```python
from build123d import *

# Parameters (mm, degrees)
SKETCH1_R           = 19.075
SKETCH1_R_2         = 2.675
BOSS_EXTRUDE1_DEPTH = 2.54
BOSS_EXTRUDE2_START = -2.54
SKETCH2_R           = 2.675
SKETCH2_R_2         = 2
BOSS_EXTRUDE2_DEPTH = 2.54
CUT_EXTRUDE1_DEPTH  = 43.502371699


with BuildPart() as part:
    # Sketch1 → Boss-Extrude1 (new body)
    with BuildSketch(Plane(origin=(0, 0, 0), x_dir=(0, 0, -1), z_dir=(1, 0, 0))):
        with BuildLine():
            Line((-30, 26.457513111), (-30, -26.457513111))
            ThreePointArc((-30, -26.457513111), (-28.284271247, -28.284271247), (-26.457513111, -30))
            Line((-26.457513111, -30), (26.457513111, -30))
            ThreePointArc((26.457513111, -30), (28.284271247, -28.284271247), (30, -26.457513111))
            Line((30, -26.457513111), (30, 26.457513111))
            ThreePointArc((30, 26.457513111), (28.284271247, 28.284271247), (26.457513111, 30))
            Line((26.457513111, 30), (-26.457513111, 30))
            ThreePointArc((-26.457513111, 30), (-28.284271247, 28.284271247), (-30, 26.457513111))
        make_face()
        Circle(SKETCH1_R, mode=Mode.SUBTRACT)
        with Locations((-23.425, -23.425)):
            Circle(SKETCH1_R_2, mode=Mode.SUBTRACT)
        with Locations((23.425, -23.425)):
            Circle(SKETCH1_R_2, mode=Mode.SUBTRACT)
        with Locations((23.425, 23.425)):
            Circle(SKETCH1_R_2, mode=Mode.SUBTRACT)
        with Locations((-23.425, 23.425)):
            Circle(SKETCH1_R_2, mode=Mode.SUBTRACT)
    extrude(amount=BOSS_EXTRUDE1_DEPTH)

    # Sketch2 → Boss-Extrude2 (add)
    # profile 1 of 4: a face of its own
    with BuildSketch(Plane(origin=(2.54, 0, 0), x_dir=(0, 0, -1), z_dir=(1, 0, 0)).offset(BOSS_EXTRUDE2_START)):
        with Locations((-23.425, -23.425)):
            Circle(SKETCH2_R)
        with Locations((-23.425, -23.425)):
            Circle(SKETCH2_R_2, mode=Mode.SUBTRACT)
    # profile 2 of 4: a face of its own
    with BuildSketch(Plane(origin=(2.54, 0, 0), x_dir=(0, 0, -1), z_dir=(1, 0, 0)).offset(BOSS_EXTRUDE2_START)):
        with Locations((23.425, 23.425)):
            Circle(SKETCH2_R)
        with Locations((23.425, 23.425)):
            Circle(SKETCH2_R_2, mode=Mode.SUBTRACT)
    # profile 3 of 4: a face of its own
    with BuildSketch(Plane(origin=(2.54, 0, 0), x_dir=(0, 0, -1), z_dir=(1, 0, 0)).offset(BOSS_EXTRUDE2_START)):
        with Locations((23.425, -23.425)):
            Circle(SKETCH2_R)
        with Locations((23.425, -23.425)):
            Circle(SKETCH2_R_2, mode=Mode.SUBTRACT)
    # profile 4 of 4: a face of its own
    with BuildSketch(Plane(origin=(2.54, 0, 0), x_dir=(0, 0, -1), z_dir=(1, 0, 0)).offset(BOSS_EXTRUDE2_START)):
        with Locations((-23.425, 23.425)):
            Circle(SKETCH2_R)
        with Locations((-23.425, 23.425)):
            Circle(SKETCH2_R_2, mode=Mode.SUBTRACT)
    extrude(amount=BOSS_EXTRUDE2_DEPTH)

    # Sketch3 → Cut-Extrude1 (cut, through all)
    with BuildSketch(Plane(origin=(2.54, 0, 0), x_dir=(0, 0, -1), z_dir=(1, 0, 0))):
        Polygon((-14.125, 30), (-14.125, 12.819516372), (16.436338552, -9.68), (30, -9.68), (30, 30), align=None)
    extrude(amount=-CUT_EXTRUDE1_DEPTH, mode=Mode.SUBTRACT)


solid = part.part
```
The model under review builds one solid part; all positions refer to its coordinate system, in mm. A direction names the side the tool comes from. Round coordinates to 2 decimals unless told otherwise and drop trailing zeros. Write each loop counter-clockwise with the first axis right and the second up, starting at its lowest first coordinate (ties: lowest second). Pieces come first, ordered by that corner, then holes.
(1) We need section B-B on x = 2.15. Give the boundary of the cut face in (y, z) (3 decimals).
(2) We need section A-A on y = 22.5. Give the boundary of the cut face in (x, z) (3 decimals), and give its area (3 significant figures).
(3) We need section D-D on y = 0. Give the boundary of the cut face in (x, z) (3 decimals), and give its area (3 significant figures).
(4) Mouldability with a two-part tool opening along Z and no side actions: class faces 3 (the cylindrical face through (1.25, -28.26, 28.31)), 4 (the cylindrical face through (1.25, -15.09, 11.67)), 5 (the flat face through (1, 22, 14.125)), 6 (the flat face through (0, -20, 7)) as +Z half, -Z half, draft (parallel to the pull), parting line (faces both ways), or undercut.
(5) Wall thickness on L1, parallel to Z at x = 1.7, y = 21 (3 decimals); L2, parallel to Y at x = 1.7, z = 23; L3, parallel to Y at x = 0.4, z = -16.5: over which ranges is each line inside the solid? List them lowest first.
(6) Machinability: for faces 1 (the flat face through (1, -9.68, -23)), 2 (the cylindrical face through (1.25, 25.11, 22.35)), which of the approach directions +Z, -Z, +X, -X, +Y, -Y give a long, thin tool a straight path to every point of the face, cutting with its end or side? Answer none if there is none.
(7) Insertion check: pin 1 (3 mm diameter, centred on y = 23.425, z = 23.425, fed in from +X); pin 2 (0.8 mm diameter, centred on x = 1, z = -25, fed in from +Y). Each pin has a flat end and moves straight along its axis. Give the tip position at first contact, or say it passes through.
(8) We need section C-C on z = 0. Give the boundary of the cut face in (x, y) (3 decimals).
Findings below:
1. outline: (-30, -26.458) arc R40 ccw to (-26.458, -30) - (-9.68, -30) - (-9.68, -16.436) arc R19.075 cw (long way) to (12.82, 14.125) - (30, 14.125) - (30, 26.458) arc R40 ccw to (26.458, 30) - (-26.458, 30) arc R40 ccw to (-30, 26.458) - close; hole circle Ø4 at (-23.425, -23.425); hole circle Ø4 at (-23.425, 23.425); hole circle Ø4 at (23.425, 23.425)
2. outline: (0, 14.125) - (2.54, 14.125) - (2.54, 21.652) - (0, 21.652) - close; (0, 25.198) - (2.54, 25.198) - (2.54, 30) - (0, 30) - close
2. area: 31.3 mm2
3. outline: (0, 19.075) - (2.54, 19.075) - (2.54, 30) - (0, 30) - close
3. area: 27.7 mm2
4. face 3: +Z half
4. face 4: undercut
4. face 5: -Z half
4. face 6: draft
5. L1: z = 14.125 to 30
5. L2: y = -30 to -25.38, -21.47 to 21.47, 25.38 to 30
5. L3: y = -30 to -9.68
6. face 1: -Z, +X, -X, +Y
6. face 2: +X, -X
7. pin 1: passes through
7. pin 2: stops at y = -9.68
8. outline: (0, -30) - (2.54, -30) - (2.54, -19.075) - (0, -19.075) - close
